Could you check a few things on this drawing? It's one solid part, dimensions in mm from its lowest x, y, z. A direction names the side the tool comes from. Give positions to 0.01 mm unless a question says otherwise; leave off trailing zeros. Write each loop counter-clockwise with the first axis right and the second up, starting at its lowest first coordinate (ties: lowest second). Pieces come first, ordered by that corner, then holes. Notation, with made-up numbers: (70, -9.75) -> (120, -9.75) arc R13 cw to (120, 2.25) -> close; hole circle Ø1 at (35, 82). An arc over 180 degrees is marked (long way). Use CSV: the item, a comma, the result in double quotes. Start each with the question number.
(1) Suppose I cut it at C-C on x = 19. List the corners of the cut face in (y, z) for me, plus the area to 3 significant figures.
(2) For pin 1 Ø7 at (x, z) = (20, 10) entering from -Y; pin 2 Ø5 at (y, z) = (16.5, 10.5) entering from +X; pin 3 Ø7.5 at (x, y) = (6.5, 16.5) entering from +Z, each with a flat end and sliding along its axis, tell me the tip position at first contact or that it passes through.
(3) If we mould it in two halves opening along X, with no side actions, what happens to the marked faces 1, 2 and 3? For each: pulls with the +X half, pulls with the -X half, needs draft (parallel to the pull), parting line crosses it, or undercut.
(4) Which directions (+Z, -Z, +X, -X, +Y, -Y) give clear straight access to the entire face, cutting with the end or side of a thin tool? Please do the marked faces 4, 5 and 6.
(5) I need wall thicknesses on L1, parallel to Z at x = 17.5, y = 16; L2, parallel to Y at x = 6.5, z = 8; L3, parallel to Y at x = 20.5, z = 6.5. Which ranges of each line are inside material? Lowest first, please. Write a range as [from, to].
(6) Suppose I cut it at B-B on z = 8.75. List the corners of the cut face in (x, y) for me, plus the area to 3 significant figures.
(7) Suppose I cut it at D-D on y = 29.5. List the corners of the cut face in (x, z) for me.
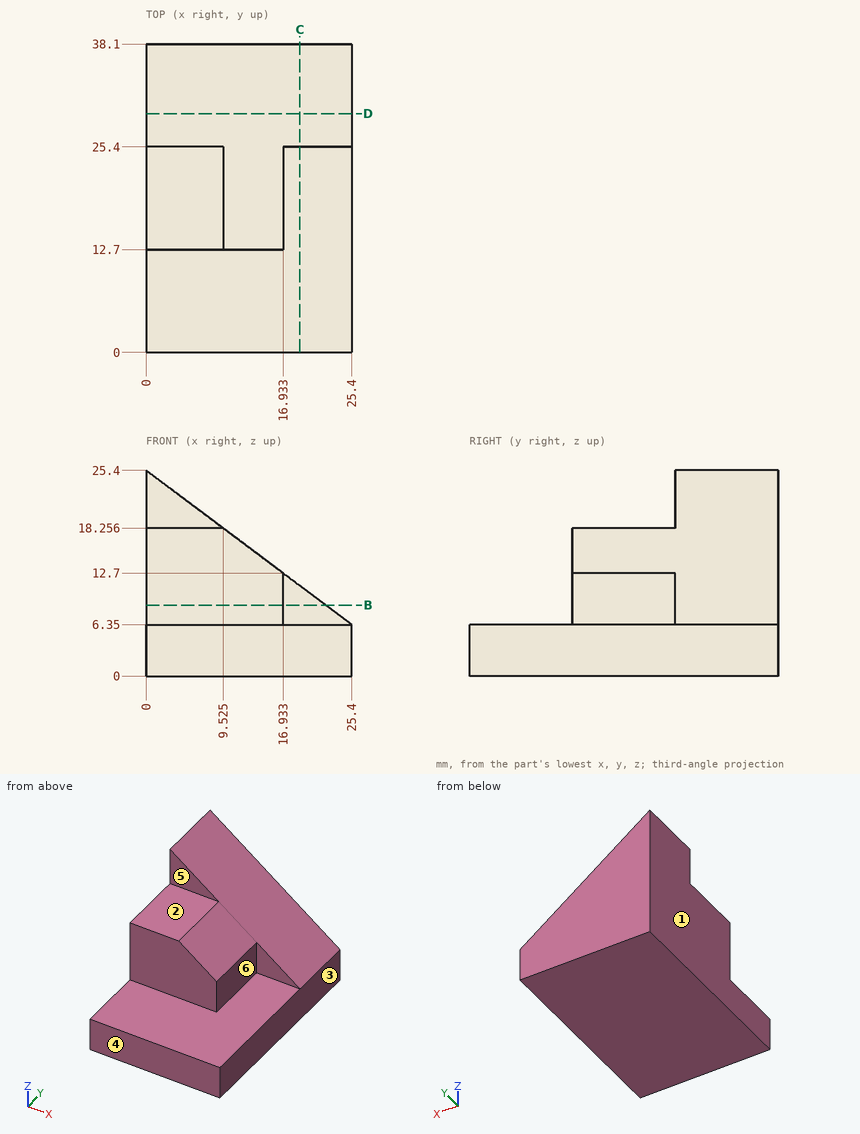
Geometry says:
1,outline,"(0, 0) -> (38.1, 0) -> (38.1, 11.15) -> (25.4, 11.15) -> (25.4, 6.35) -> (0, 6.35) -> close"
1,area,"303 mm²"
2,pin 1,"y = 12.7"
2,pin 2,"x = 16.93"
2,pin 3,"z = 18.26"
3,face 1,"pulls with the -X half"
3,face 2,"needs draft"
3,face 3,"pulls with the +X half"
4,face 4,"+Z, -Z, +X, -X, -Y"
4,face 5,"+Z, +X, -X, -Y"
4,face 6,"+Z, +X, -Y"
5,L1,"[0, 6.35]"
5,L2,"[12.7, 38.1]"
5,L3,"[25.4, 38.1]"
6,outline,"(0, 12.7) -> (16.93, 12.7) -> (16.93, 25.4) -> (22.2, 25.4) -> (22.2, 38.1) -> (0, 38.1) -> close"
6,area,"497 mm²"
7,outline,"(0, 0) -> (25.4, 0) -> (25.4, 6.35) -> (0, 25.4) -> close"
